from build123d import *

# Parameters (mm, degrees)
F0_W     = 44.45
F0_H     = 25.4
F1_DEPTH = 12.7
F4_D     = 8.3312
F4_DEPTH = 12.7
F4_TIP   = 2.5029449946
F5_D     = 8.3312
F5_DEPTH = 12.7
F5_TIP   = 2.5029449946
F6_D     = 4.318
F6_DEPTH = 9.525
F6_TIP   = 1.2972580765
F7_D     = 11.1125


with BuildPart() as f1:
    # F0 (on Front) → F1 (new body, symmetric)
    with BuildSketch(Plane.XZ):
        Rectangle(F0_W, F0_H)
    extrude(amount=F1_DEPTH, both=True)

    # F4
    with Locations(Plane.XY.offset(12.7)):
        with Locations((-9.525, 0)):
            Hole(F4_D / 2, depth=F4_DEPTH)
            with Locations((0, 0, -(F4_DEPTH + F4_TIP / 2))):  # 118° drill point
                Cone(0, F4_D / 2, F4_TIP, mode=Mode.SUBTRACT)

    # F5
    with Locations(Plane.XY.offset(12.7)):
        with Locations((9.525, 0)):
            Hole(F5_D / 2, depth=F5_DEPTH)
            with Locations((0, 0, -(F5_DEPTH + F5_TIP / 2))):  # 118° drill point
                Cone(0, F5_D / 2, F5_TIP, mode=Mode.SUBTRACT)

    # F6
    with Locations(Plane.XY.offset(12.7)):
        with Locations((0, 8.89), (0, -8.89)):
            Hole(F6_D / 2, depth=F6_DEPTH)
            with Locations((0, 0, -(F6_DEPTH + F6_TIP / 2))):  # 118° drill point
                Cone(0, F6_D / 2, F6_TIP, mode=Mode.SUBTRACT)

    # F7 (through all)
    with Locations(Plane.YZ.offset(22.225)):
        with Locations((0, 0)):
            Hole(F7_D / 2)


solid = f1.part
The model under review builds one solid part; all positions refer to its coordinate system, in mm. A direction names the side the tool comes from. Round coordinates to 2 decimals unless told otherwise and drop trailing zeros. Order: outer loops, then holes, each group sorted by start corner. A loop starts at its lowest first (then second) coordinate and runs counter-clockwise, first axis right, second up. Notation, with made-up numbers: (68.5, 76.25) - (99.5, 76.25) arc R20 cw to (99.5, 107.25) - close; hole circle Ø7 at (29, 77). An arc over 180 degrees is marked (long way). Use one line per item in the form item = value.
Q1. Add section B-B on x = 19. Give the boundary of the cut face in (y, z), then the cut area to 3 significant figures.
Response values:
outline = (-12.7, -12.7) - (12.7, -12.7) - (12.7, 12.7) - (-12.7, 12.7) - close; hole circle Ø11.11 at (0, 0)
area = 548 mm^2
Q2. Add section A-A on y = 0. Give the boundary of the cut face in (x, z) (3 decimals), then the cut area to 3 significant figures.
Response values:
outline = (-22.225, -12.7) - (22.225, -12.7) - (22.225, -5.556) - (-22.225, -5.556) - close; (-22.225, 5.556) - (-13.691, 5.556) - (-13.691, 12.7) - (-22.225, 12.7) - close; (-5.359, 5.556) - (5.359, 5.556) - (5.359, 12.7) - (-5.359, 12.7) - close; (13.691, 5.556) - (22.225, 5.556) - (22.225, 12.7) - (13.691, 12.7) - close
area = 516 mm^2
Q3. Add section C-C on y = -4.75. Give the boundary of the cut face in (x, z) (3 decimals).
Response values:
outline = (-22.225, -12.7) - (22.225, -12.7) - (22.225, -2.883) - (-22.225, -2.883) - close; (-22.225, 2.883) - (22.225, 2.883) - (22.225, 12.7) - (-22.225, 12.7) - close
Q4. Tool access review of faces 5 (the cylindrical face through (-5.363, 0.183, 9.128)), 6 (the flat face through (0, 12.7, 0)): name each direction out of +Z, -Z, +X, -X, +Y, -Y from which nothing blocks a thin tool from reaching the whole face with its end or side.
Response values:
face_5 = +Z
face_6 = +Z, -Z, +X, -X, +Y
Q5. Mouldability with a two-part tool opening along Z and no side actions: class faces 1 (the flat face through (0, 0, -12.7)), 2 (the cylindrical face through (0.28, 11.03, 7.87)), 3 (the conical face through (-0.3, 9.1, 2.1)), 4 (the cylindrical face through (-0.311, 1.204, -5.424)) as pulls with the +Z half, pulls with the -Z half, needs draft (parallel to the pull), parting line crosses it, or undercut.
Response values:
face_1 = pulls with the -Z half
face_2 = needs draft
face_3 = pulls with the +Z half
face_4 = undercut
Q6. Clearance check with a flat-ended pin moving along its axis: P1, Ø7.5, axis at x = -9.525, y = 0, coming from the +Z side. State where the tip first meets the part, or that it passes through.
Response values:
P1 = -4.1
Q7. To check wall thickness, follow line 1 (Y direction, x = 0, z = 7.25); line 2 (X direction, y = 0, z = 10.5) (3 decimals); line 3 (Z direction, x = 5, y = -1.5). State the ranges of each line that lie inside material, in increasing order.
Response values:
line_1 = -12.7 to -11.05, -6.73 to 6.73, 11.05 to 12.7
line_2 = -22.225 to -13.691, -5.359 to 5.359, 13.691 to 22.225
line_3 = -12.7 to -5.35, 5.35 to 12.7
Q8. Add section D-D on x = 11. Give the boundary of the cut face in (y, z), then the cut area to 3 significant figures.
Response values:
outline = (-12.7, -12.7) - (12.7, -12.7) - (12.7, 12.7) - (3.9, 12.7) - (3.9, 3.96) arc R5.56 cw (long way) to (-3.9, 3.96) - (-3.9, 12.7) - (-12.7, 12.7) - close
area = 489 mm^2
